Job drawing, mm, ordinate dimensions from the low corner. One solid piece. A direction names the side the tool comes from. Give positions to 0.01 mm unless a question says otherwise; leave off trailing zeros. Order: outer loops, then holes, each group sorted by start corner. A loop starts at its lowest first (then second) coordinate and runs counter-clockwise, first axis right, second up.
Item 1: Band-saw the part on D-D on z = 47.5. Give the cut face in (x, y), plus the area to 3 significant figures.
Item 2: Two-plate mould, pull along X, no slides. Class the marked faces 3, 4 and 5: released by +X, released by -X, zero draft, split by the parting line, or undercut.
Item 3: Band-saw the part on B-B on x = 20.05. Give the cut face in (y, z), plus the area to 3 significant figures.
Item 4: Which spindle directions (+Z, -Z, +X, -X, +Y, -Y) get a long thin tool onto all of the face, cutting with end or side? Do the marked faces 1 and 2. Say none if no direction does.
Item 5: Band-saw the part on C-C on y = 5. Give the cut face in (x, z), plus the area to 3 significant figures.
Item 6: Flat gauge pins, fed straight in: P1, Ø10, axis at x = 14, z = 39.5, coming from the -Y side; P2, Ø4.5, axis at x = 34.5, y = 9, coming from the +Z side; P3, Ø8, axis at x = 14, y = 7.5, coming from the -Z side. Where does each tip first touch, or does it go through?
Item 7: Wall check: L1, parallel to Y at x = 33.7, z = 0.4; L2, parallel to Z at x = 20.05, y = 10; L3, parallel to Z at x = 7.5, y = 6.25. Give the ranges that are in metal, low to high.
Item 8: Band-saw the part on A-A on x = 33.7. Give the cut face in (y, z).
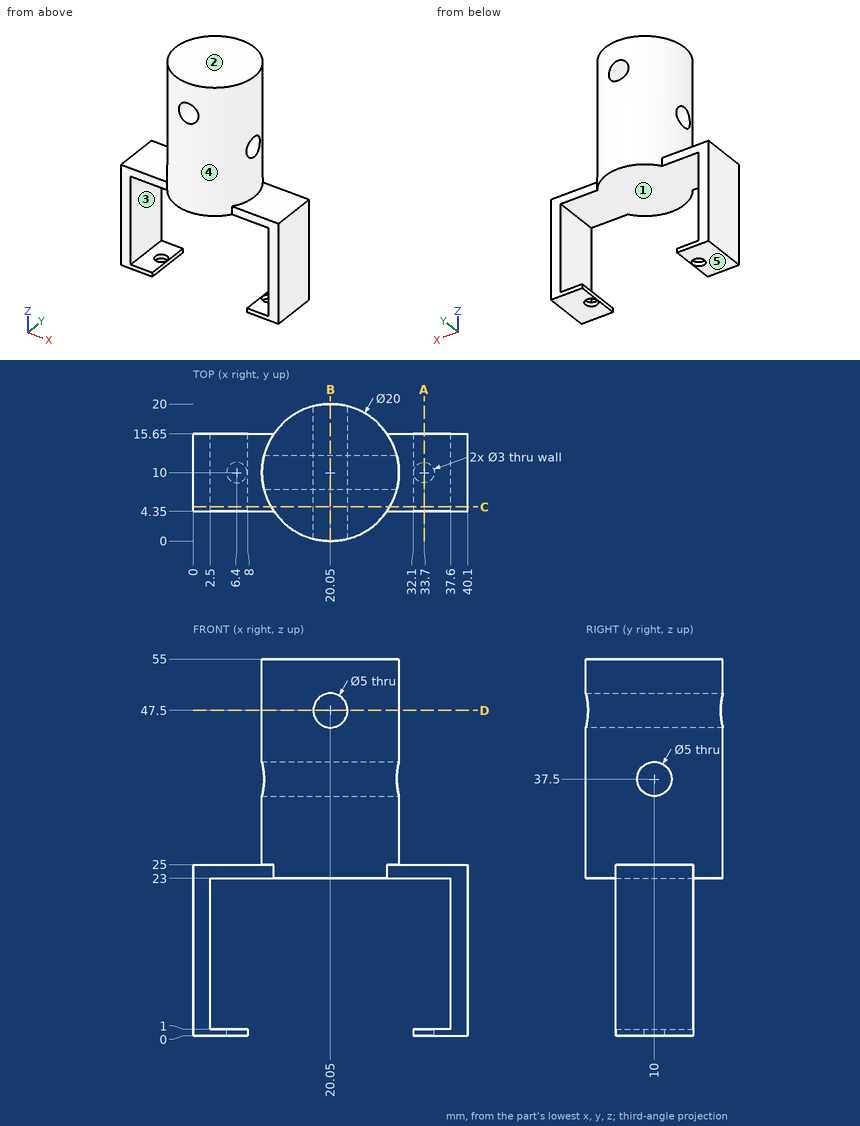
The answers:
1. outline: (17.55, 0.32) - (17.55, 19.68) arc R10 ccw to start; (22.55, 0.32) arc R10 ccw to (22.55, 19.68) - close
1. area: 215 mm2
2. face 3: undercut
2. face 4: split by the parting line
2. face 5: zero draft
3. outline: (0, 23) - (20, 23) - (20, 45) - (0, 45) - close; (0, 50) - (20, 50) - (20, 55) - (0, 55) - close; hole circle Ø5 at (10, 37.5)
3. area: 520 mm2
4. face 1: +Y, -Y
4. face 2: +Z, +X, -X, +Y, -Y
5. outline: (0, 0) - (8, 0) - (8, 1) - (2.5, 1) - (2.5, 23) - (37.6, 23) - (37.6, 1) - (32.1, 1) - (32.1, 0) - (40.1, 0) - (40.1, 25) - (28.71, 25) - (28.71, 55) - (11.39, 55) - (11.39, 25) - (0, 25) - close; hole circle Ø5 at (20.05, 47.5)
5. area: 706 mm2
6. P1: stops at y = 0.06
6. P2: stops at z = 25
6. P3: stops at z = 23
7. L1: y = 4.35 to 8.5, 11.5 to 15.65
7. L2: z = 23 to 35, 40 to 45, 50 to 55
7. L3: z = 0 to 1, 23 to 25
8. outline: (4.35, 0) - (8.5, 0) - (8.5, 1) - (4.35, 1) - close; (4.35, 23) - (15.65, 23) - (15.65, 25) - (4.35, 25) - close; (11.5, 0) - (15.65, 0) - (15.65, 1) - (11.5, 1) - close
